Design review of the part built by this model. Coordinates are the model's own, in mm. Round coordinates to 2 decimals unless told otherwise and drop trailing zeros. Order: outer loops, then holes, each group sorted by start corner. A loop starts at its lowest first (then second) coordinate and runs counter-clockwise, first axis right, second up. Notation, with made-up numbers: M 31,-31 L 88,-31 A22 ccw 88,6 Z; hole C 45.25,84 d10. An arc over 180 degrees is marked long. Write item = value, one per line. Start each with the question number.
```python
from build123d import *

# Parameters (mm, degrees)
AUFSATZ_LINEAR_AUSTRAGEN1_DEPTH = 10
FASE1_SIZE                      = 10


with BuildPart() as part:
    # Skizze1 → Aufsatz-Linear austragen1 (new body)
    with BuildSketch(Plane.XY):
        Polygon((-434.714346895, -88.5), (-434.714346895, 88.5), (0, 85), (0, -85), align=None)
    extrude(amount=AUFSATZ_LINEAR_AUSTRAGEN1_DEPTH)

    # Fase1
    fase1_edges = [part.edges().sort_by_distance(p)[0] for p in [
        (-434.714346895, 0, 10),
        (-217.357173448, 86.75, 10),
        (0, 0, 10),
        (-217.357173448, -86.75, 10),
    ]]
    chamfer(fase1_edges, length=FASE1_SIZE - 0.0001)  # a hair under: the kernel refuses the full size


solid = part.part
```
(1) Consider section C-C, the plane z = 4.5. Write out the cut boundary in (x, y), then the cut area to 3 significant figures.
(2) Insertion check: pin 1 (4 mm diameter, centred on y = -53, z = 8.5, fed in from -X); pin 2 (2 mm diameter, centred on y = 55, z = 8.5, fed in from +X); pin 3 (5 mm diameter, centred on x = -105, z = 3, fed in from +Y). Each pin has a flat end and moves straight along its axis. Give the tip position at first contact, or say it passes through.
(3) For line 1 along Y through (x, z) = (-149, 8); line 2 along X through (y, z) = (41, 6.5); line 3 along Y through (x, z) = (-110.5, 1.5), list the stretches that pass through material, from the lowest coordinate up. Write a range as [from, to].
Completed:
q1.outline = M -430.21,-83.96 L -4.5,-80.54 L -4.5,80.54 L -430.21,83.96 Z
q1.area = 70,000 mm2
q2.pin_1 = -428.21
q2.pin_2 = -7.5
q2.pin_3 = 85.35
q3.line_1 = [-78.2, 78.2]
q3.line_2 = [-428.21, -6.5]
q3.line_3 = [-84.39, 84.39]
